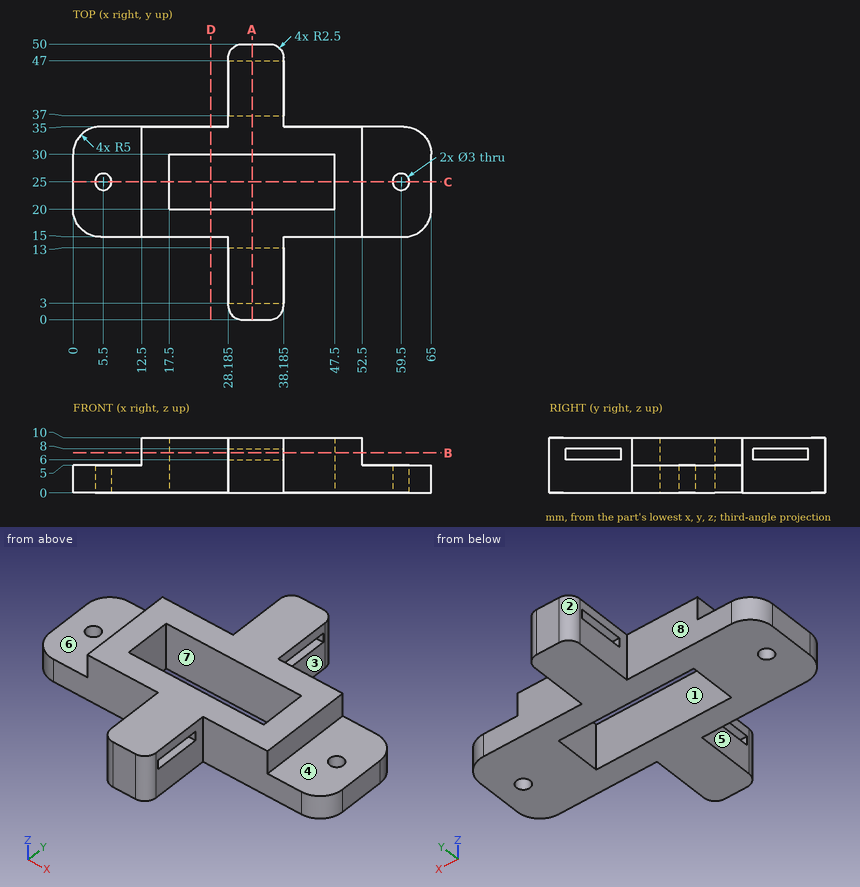
Drawing for the job (mm, zero at the part's lowest x, y, z). A direction names the side the tool comes from. Round coordinates to 2 decimals unless told otherwise and drop trailing zeros. Write each loop counter-clockwise with the first axis right and the second up, starting at its lowest first coordinate (ties: lowest second). Pieces come first, ordered by that corner, then holes. Notation, with made-up numbers: (73, 64) - (80, 64) arc R19 ccw to (80, 94) - close; hole circle Ø11 at (-27, 65). An arc over 180 degrees is marked (long way). Return JSON: item names as keys, results as strings. Group by question number.
Item 1: Flat gauge pins, fed straight in: pin 1 Ø5 at (x, z) = (28, 8.5) entering from +Y; pin 2 Ø1 at (y, z) = (29.5, 8) entering from -X; pin 3 Ø1 at (y, z) = (27.5, 8) entering from +X; pin 4 Ø8 at (x, y) = (46.5, 30) entering from -Z. Where does each tip first touch, or does it go through?
Item 2: Mould opens along Y. For the marked faces 1, 2 and 3 say: +Y half, -Y half, draft (parallel to the pull), parting line (faces both ways), or undercut.
Item 3: Band-saw the part on B-B on z = 7.25. List the corners of the cut face in (x, y) (3 decimals), plus the area to 3 significant figures.
Item 4: Band-saw the part on A-A on x = 32.5. List the corners of the cut face in (y, z).
Item 5: Probe probe 1 along X at (y, z) = (21.5, 8.75); probe 2 along Y at (x, z) = (59.5, 2.05); probe 3 along Y at (x, z) = (25.5, 7.5). List the from-to ranges inside material, lowest first.
Item 6: Band-saw the part on C-C on y = 25. List the corners of the cut face in (x, z).
Item 7: Band-saw the part on D-D on x = 25. List the corners of the cut face in (y, z).
Item 8: 3-axis set-ups, long thin cutter, end or side, ignore diameter. For the marked faces 4, 5, 6, 7 and 8: which of +Z, -Z, +X, -X, +Y, -Y reach the whole face in a straight line?
Resolved:
{
 "1": {"pin 1": "stops at y = 49.99", "pin 2": "stops at x = 12.5", "pin 3": "stops at x = 52.5", "pin 4": "stops at z = 0"},
 "2": {"face 1": "undercut", "face 2": "+Y half", "face 3": "draft"},
 "3": {"outline": "(12.5, 15) - (28.185, 15) - (28.185, 13) - (38.185, 13) - (38.185, 15) - (52.5, 15) - (52.5, 35) - (38.185, 35) - (38.185, 37) - (28.185, 37) - (28.185, 35) - (12.5, 35) - close; (28.185, 2.5) arc R2.5 ccw to (30.685, 0) - (35.685, 0) arc R2.5 ccw to (38.185, 2.5) - (38.185, 3) - (28.185, 3) - close; (28.185, 47) - (38.185, 47) - (38.185, 47.5) arc R2.5 ccw to (35.685, 50) - (30.685, 50) arc R2.5 ccw to (28.185, 47.5) - close; hole (17.5, 20) - (47.5, 20) - (47.5, 30) - (17.5, 30) - close", "area": "595 mm²"},
 "4": {"outline": "(0, 0) - (20, 0) - (20, 10) - (0, 10) - close; (30, 0) - (50, 0) - (50, 10) - (30, 10) - close; hole (3, 6) - (13, 6) - (13, 8) - (3, 8) - close; hole (37, 6) - (47, 6) - (47, 8) - (37, 8) - close"},
 "5": {"probe 1": "x = 12.5 to 17.5, 47.5 to 52.5", "probe 2": "y = 15 to 23.5, 26.5 to 35", "probe 3": "y = 15 to 20, 30 to 35"},
 "6": {"outline": "(0, 0) - (4, 0) - (4, 5) - (0, 5) - close; (7, 0) - (17.5, 0) - (17.5, 10) - (12.5, 10) - (12.5, 5) - (7, 5) - close; (47.5, 0) - (58, 0) - (58, 5) - (52.5, 5) - (52.5, 10) - (47.5, 10) - close; (61, 0) - (65, 0) - (65, 5) - (61, 5) - close"},
 "7": {"outline": "(15, 0) - (20, 0) - (20, 10) - (15, 10) - close; (30, 0) - (35, 0) - (35, 10) - (30, 10) - close"},
 "8": {"face 4": "+Z, +X, +Y, -Y", "face 5": "+Z, -Z, -X, -Y", "face 6": "+Z, -X, +Y, -Y", "face 7": "+Z, -Z", "face 8": "+Z, -Z, -X, +Y"}
}
